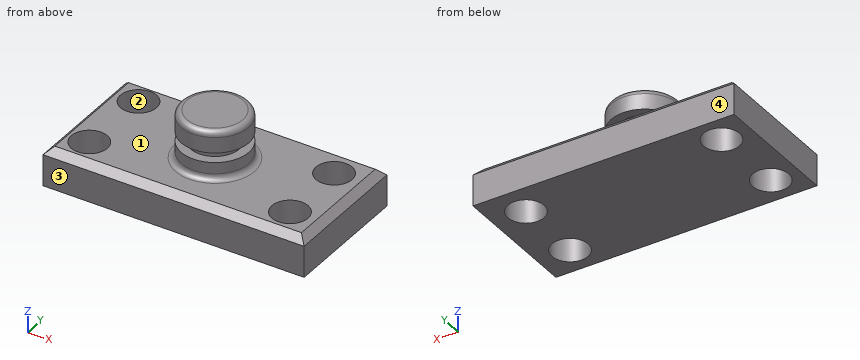
from build123d import *

# Parameters (mm, degrees)
F0_W     = 137.63725
F0_H     = 68.484548
F1_DEPTH = 20.32
F2_R     = 9.525
F3_DEPTH = 25.4
F4_W     = 17.78
F4_H     = 25.4
F6_W     = 5.08
F6_H     = 5.08
F8_SIZE  = 3.81
F9_R     = 3.048


with BuildPart() as f1:
    # F0 (on Top) → F1 (new body)
    with BuildSketch(Plane.XY):
        Rectangle(F0_W, F0_H)
    extrude(amount=F1_DEPTH)

    # F2 (on face) → F3 (cut)
    with BuildSketch(Plane.XY.offset(20.32)):
        with Locations((51.390208, 17.808059)):
            Circle(F2_R)
        with Locations((-53.108271, 20.035554)):
            Circle(F2_R)
        with Locations((-53.903826, -19.373486)):
            Circle(F2_R)
        with Locations((51.681355, -19.040003)):
            Circle(F2_R)
    extrude(amount=-F3_DEPTH, mode=Mode.SUBTRACT)

    # F4 (on Front) → F5 (revolve)
    with BuildSketch(Plane.XZ):
        with Locations((8.89, 33.02)):
            Rectangle(F4_W, F4_H)
    revolve(axis=Axis((0, 0, 33.02), (0, 0, 1)))

    # F6 (on Front) → F7 (revolve, cut)
    with BuildSketch(Plane.XZ):
        with Locations((15.342483, 31.907923)):
            Rectangle(F6_W, F6_H)
    revolve(axis=Axis((0, 0, 43.360371), (0, 0, -1)), mode=Mode.SUBTRACT)

    # F8
    f8_edges = [f1.edges().sort_by_distance(p)[0] for p in [
        (0, -34.242274, 20.32),
        (0, 34.242274, 20.32),
        (68.818625, 0, 20.32),
        (-68.818625, 0, 20.32),
    ]]
    chamfer(f8_edges, length=F8_SIZE)

    # F9
    f9_edges = [f1.edges().sort_by_distance(p)[0] for p in [
        (-17.78, 0, 45.72),
        (-17.78, 0, 20.32),
    ]]
    fillet(f9_edges, radius=F9_R)


solid = f1.part
Geometry: final body of the model. Coordinates: model frame, mm. Face numbers are marked on the shaded views. Give positions to 0.01 mm unless a question says otherwise; leave off trailing zeros. Write each loop counter-clockwise with the first axis right and the second up, starting at its lowest first coordinate (ties: lowest second). Pieces come first, ordered by that corner, then holes. Notation, with made-up numbers: (-17, -32.5) -> (23, -32.5) arc R17 ccw to (23, -20.5) -> close; hole circle Ø4 at (16, 11). An arc over 180 degrees is marked (long way). Answer as a JSON object with one key per item and string values.
1. Cut plane B-B on z = 3. Output: boundary loops of the cut face in (x, y) (3 decimals).
Ans:
{"outline": "(-68.819, -34.242) -> (68.819, -34.242) -> (68.819, 34.242) -> (-68.819, 34.242) -> close; hole circle Ø19.05 at (-53.904, -19.373); hole circle Ø19.05 at (-53.108, 20.036); hole circle Ø19.05 at (51.39, 17.808); hole circle Ø19.05 at (51.681, -19.04)"}
2. Cut plane A-A on y = 0. Output: boundary loops of the cut face in (x, z), and give its area (3 significant figures).
Ans:
{"outline": "(-68.82, 0) -> (68.82, 0) -> (68.82, 16.51) -> (65.01, 20.32) -> (20.83, 20.32) arc R3.05 cw to (17.78, 23.37) -> (17.78, 29.37) -> (12.8, 29.37) -> (12.8, 34.45) -> (17.78, 34.45) -> (17.78, 42.67) arc R3.05 ccw to (14.73, 45.72) -> (-14.73, 45.72) arc R3.05 ccw to (-17.78, 42.67) -> (-17.78, 34.45) -> (-12.8, 34.45) -> (-12.8, 29.37) -> (-17.78, 29.37) -> (-17.78, 23.37) arc R3.05 cw to (-20.83, 20.32) -> (-65.01, 20.32) -> (-68.82, 16.51) -> close", "area": "3,630 mm^2"}
3. Cut plane D-D on x = -57. Output: boundary loops of the cut face in (y, z), and give its area (3 significant figures).
Ans:
{"outline": "(-34.24, 0) -> (-28.38, 0) -> (-28.38, 20.32) -> (-30.43, 20.32) -> (-34.24, 16.51) -> close; (-10.37, 0) -> (11.34, 0) -> (11.34, 20.32) -> (-10.37, 20.32) -> close; (28.73, 0) -> (34.24, 0) -> (34.24, 16.51) -> (30.43, 20.32) -> (28.73, 20.32) -> close", "area": "658 mm^2"}
4. Mould query, pull axis Y, two halves, no side actions, for the marked faces 1, 2, 3 and 4. Classes: pulls with the +Y half, pulls with the -Y half, needs draft (parallel to the pull), parting line crosses it, or undercut.
Ans:
{"face 1": "needs draft", "face 2": "undercut", "face 3": "pulls with the -Y half", "face 4": "pulls with the +Y half"}
5. Contact query for flat-ended pins moving along their axis: pin 1 (4 mm diameter, centred on x = 18.5, y = 19, fed in from +Z); pin 2 (3 mm diameter, centred on x = -15, z = 34.5, fed in from -Y). Output: stop coordinate, or through.
Ans:
{"pin 1": "stops at z = 20.32", "pin 2": "stops at y = -11.57"}
6. Cut plane C-C on x = -33.5. Output: boundary loops of the cut face in (y, z), and give its area (3 significant figures).
Ans:
{"outline": "(-34.24, 0) -> (34.24, 0) -> (34.24, 16.51) -> (30.43, 20.32) -> (-30.43, 20.32) -> (-34.24, 16.51) -> close", "area": "1,380 mm^2"}
7. Ray query, probe 1 along X at (y, z) = (-12, 11); probe 2 along Y at (x, z) = (56.5, 9); probe 3 along Y at (x, z) = (45, 10). Return the intervals inside material, ascending. Write a range as from..to.
Ans:
{"probe 1": "x = -68.82..-59.93, -47.87..45.27, 58.1..68.82", "probe 2": "y = -34.24..-27.26, -10.82..9.77, 25.85..34.24", "probe 3": "y = -34.24..-25.83, -12.25..10.74, 24.87..34.24"}
